Verification items for the finished model (mm, model axes). Face numbers are marked on the shaded views. Round coordinates to 2 decimals unless told otherwise and drop trailing zeros. Order: outer loops, then holes, each group sorted by start corner. A loop starts at its lowest first (then second) coordinate and runs counter-clockwise, first axis right, second up. Notation, with made-up numbers: (51.25, 35) -> (101.25, 35) arc R32 ccw to (101.25, 66) -> close; hole circle Ø5 at (-4, -1.75). An arc over 180 degrees is marked (long way). Return JSON: item names as keys, results as strings. Group by question number.
Item 1: Scan lines: probe 1 along Z at (x, y) = (0, -1.2); probe 2 along X at (y, z) = (1.9, -0.1); probe 3 along Z at (x, y) = (-0.6, -0.8). Record each from-to range of solid material in increasing order. Write a range as from..to.
Item 2: Sectioned sample at A-A on z = 1.05. Record the cut outline in (x, y).
Item 3: Sectioned sample at D-D on z = 1.6. Record the cut outline in (x, y), plus the area to 3 significant figures.
Item 4: Depth check by flat-ended pin: pin 1 Ø1.6 at (x, z) = (0, 0) entering from +Y. Enter the tip coordinate at first touch or a pass-through.
Item 5: Sectioned sample at B-B on y = -1.45. Record the cut outline in (x, z), plus the area to 3 significant figures.
Item 6: Draft check along Z on the marked faces 1, 2 and 3. Enter one of: pulls with the +Z half, pulls with the -Z half, needs draft (parallel to the pull), parting line crosses it, or undercut.
Item 7: Sectioned sample at C-C on x = -0.2. Record the cut outline in (y, z), plus the area to 3 significant figures.
Autodesk Inventor part; units mm, degrees
ref_plane "YZ Plane" through (0, 0, 0) normal (1, 0, 0) x (0, 1, 0)
ref_plane "XZ Plane" through (0, 0, 0) normal (0, 1, 0) x (-1, 0, 0)
ref_plane "XY Plane" through (0, 0, 0) normal (0, 0, 1) x (1, 0, 0)
sketch "Skizze1" plane through (0, 0, 0) normal (0, 1, 0) x (-1, 0, 0)
  line L0 (2.6558, 0) -> (1.3279, -2.3)
  line L1 (1.3279, -2.3) -> (-1.3279, -2.3)
  line L2 (-1.3279, -2.3) -> (-2.6558, 0)
  line L3 (-2.6558, 0) -> (-1.3279, 2.3)
  line L4 (-1.3279, 2.3) -> (1.3279, 2.3)
  line L5 (1.3279, 2.3) -> (2.6558, 0)
  line L6 (0, -3.22) -> (0, 3.22)
  line L7 (-3.7181, 0) -> (3.7181, 0)
  point P0 (0, 0)
  point P1 (0, 0)
  dimension "d0" = 4.6
extrude "Extrusion1" add sketch "Skizze1" along normal mid plane 5.5
sketch "Skizze2" plane through (0, 2.75, 0) normal (0, 1, 0) x (1, 0, 0)
  point P0 (0, 0)
  point P1 (0, 0)
hole "Bohrung1" at (0, 2.75, 0) direction (0, -1, 0) diameter 2.6416 end through all
properties part number "22_Hexnut_5mm" material "Messing, weicher Gelbton"
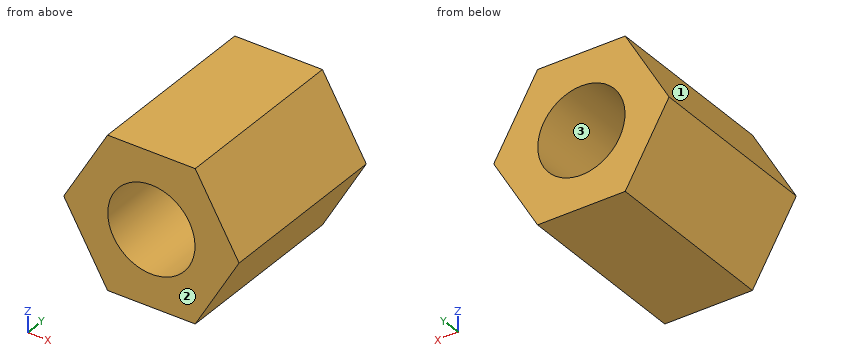
Recorded:
{
 "1": {"probe 1": "-2.3..-1.32, 1.32..2.3", "probe 2": "-2.6..-1.32, 1.32..2.6", "probe 3": "-2.3..-1.18, 1.18..2.3"},
 "2": {"outline": "(-2.05, -2.75) -> (-0.8, -2.75) -> (-0.8, 2.75) -> (-2.05, 2.75) -> close; (0.8, -2.75) -> (2.05, -2.75) -> (2.05, 2.75) -> (0.8, 2.75) -> close"},
 "3": {"outline": "(-1.73, -2.75) -> (1.73, -2.75) -> (1.73, 2.75) -> (-1.73, 2.75) -> close", "area": "19.1 mm²"},
 "4": {"pin 1": "through"},
 "5": {"outline": "(-2.66, 0) -> (-1.33, -2.3) -> (1.33, -2.3) -> (2.66, 0) -> (1.33, 2.3) -> (-1.33, 2.3) -> close; hole circle Ø2.64 at (0, 0)", "area": "12.8 mm²"},
 "6": {"face 1": "pulls with the +Z half", "face 2": "needs draft", "face 3": "undercut"},
 "7": {"outline": "(-2.75, -2.3) -> (2.75, -2.3) -> (2.75, -1.31) -> (-2.75, -1.31) -> close; (-2.75, 1.31) -> (2.75, 1.31) -> (2.75, 2.3) -> (-2.75, 2.3) -> close", "area": "10.9 mm²"}
}
